Check sheet for the drawn part. Datum: minimum x, y, z corner. Units: mm. Coordinates: 2 decimals unless noted, no trailing zeros. Order: outer loops, then holes, each group sorted by start corner. A loop starts at its lowest first (then second) coordinate and runs counter-clockwise, first axis right, second up. Notation, with made-up numbers: M 52,-27 L 85,-27 A6 cw 85,-21 Z; hole C -30.5,-13.5 d2. An arc over 180 degrees is marked long. Use one line per item in the form item = value. Start each with the question number.
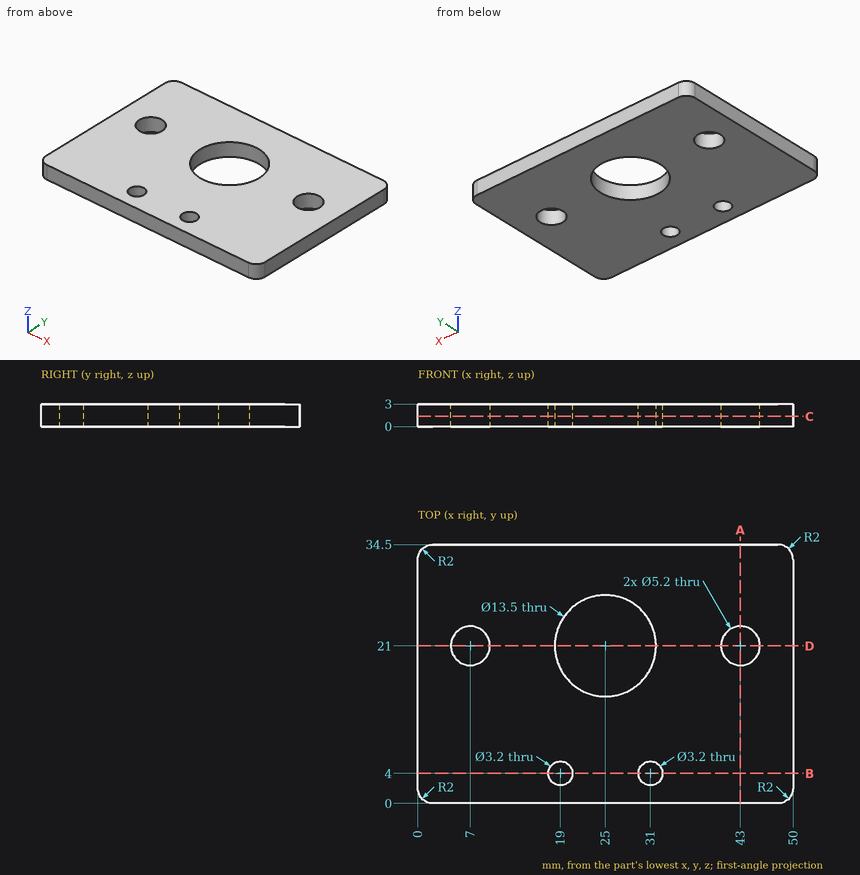
1. Cross-section at C-C on z = 1.35. Enter the section's corners in (x, y).
2. Cross-section at D-D on y = 21. Enter the section's corners in (x, z), and give its area (3 significant figures).
3. Cross-section at A-A on x = 43. Enter the section's corners in (y, z), and give its area (3 significant figures).
4. Material ranges on line 1 along Y through (x, z) = (19, 1.45); line 2 along Y through (x, z) = (43, 1.8); line 3 along Y through (x, z) = (25, 2.15), recorded low to high.
5. Cross-section at B-B on y = 4. Enter the section's corners in (x, z).
Final values:
q1.outline = M 0,2 A2 ccw 2,0 L 48,0 A2 ccw 50,2 L 50,32.5 A2 ccw 48,34.5 L 2,34.5 A2 ccw 0,32.5 Z; hole C 7,21 d5.2; hole C 19,4 d3.2; hole C 25,21 d13.5; hole C 31,4 d3.2; hole C 43,21 d5.2
q2.outline = M 0,0 L 4.4,0 L 4.4,3 L 0,3 Z; M 9.6,0 L 18.25,0 L 18.25,3 L 9.6,3 Z; M 31.75,0 L 40.4,0 L 40.4,3 L 31.75,3 Z; M 45.6,0 L 50,0 L 50,3 L 45.6,3 Z
q2.area = 78.3 mm2
q3.outline = M 0,0 L 18.4,0 L 18.4,3 L 0,3 Z; M 23.6,0 L 34.5,0 L 34.5,3 L 23.6,3 Z
q3.area = 87.9 mm2
q4.line_1 = 0 to 2.4, 5.6 to 17.91, 24.09 to 34.5
q4.line_2 = 0 to 18.4, 23.6 to 34.5
q4.line_3 = 0 to 14.25, 27.75 to 34.5
q5.outline = M 0,0 L 17.4,0 L 17.4,3 L 0,3 Z; M 20.6,0 L 29.4,0 L 29.4,3 L 20.6,3 Z; M 32.6,0 L 50,0 L 50,3 L 32.6,3 Z
